from build123d import *

# Parameters (mm, degrees)
BOSS_EXTRUDE1_DEPTH      = 6
BOSS_EXTRUDE1_DEPTH_BACK = 4
SKETCH1_R                = 2.55
SKETCH1_R_2              = 2.2
SKETCH4_W                = 10
SKETCH4_H                = 10
BOSS_EXTRUDE4_DEPTH      = 10
SKETCH5_W                = 4
SKETCH5_H                = 10
CUT_EXTRUDE1_DEPTH       = 10
BOSS_EXTRUDE5_REACH      = 54.82
SKETCH6_R                = 2
CHAMFER1_SIZE            = 2
SKETCH7_W                = 50
SKETCH7_H                = 20.5
BOSS_EXTRUDE6_DEPTH      = 10
SKETCH13_W               = 50
SKETCH13_H               = 10
BOSS_EXTRUDE9_DEPTH      = 25.5
SKETCH16_W               = 44
SKETCH16_H               = 40
CUT_EXTRUDE3_DEPTH       = 7
SKETCH17_R               = 2.6
CUT_EXTRUDE4_DEPTH       = 3
SKETCH18_W               = 2
SKETCH18_H               = 10
BOSS_EXTRUDE11_DEPTH     = 5
FILLET2_R                = 5
CUT_EXTRUDE5_REACH       = 67.666
SKETCH20_R               = 2.55
FILLET5_R                = 1.5
CUT_EXTRUDE6_DEPTH       = 3
BOSS_EXTRUDE12_START     = 2
SKETCH22_W               = 20
SKETCH22_H               = 10
BOSS_EXTRUDE12_DEPTH     = 2
CUT_EXTRUDE7_REACH       = 69.941
SKETCH23_R               = 1.6
CUT_EXTRUDE8_DEPTH       = 68.941151006


with BuildPart() as part:
    # Sketch1 → Boss-Extrude1 (new, two sides: drawn at the far end of the back side and taken through both)
    with BuildSketch(Plane.XY.offset(-BOSS_EXTRUDE1_DEPTH_BACK)):
        Polygon((-15, 0), (-15, 46), (0, 46), (0, 26), (15, 26), (15, 0), align=None)
        with Locations((-7.5, 38.5)):
            Circle(SKETCH1_R, mode=Mode.SUBTRACT)
        with Locations((7.5, 14)):
            Circle(SKETCH1_R_2, mode=Mode.SUBTRACT)
    extrude(amount=BOSS_EXTRUDE1_DEPTH + BOSS_EXTRUDE1_DEPTH_BACK)

    # Sketch4 → Boss-Extrude4 (add)
    with BuildSketch(Plane(origin=(0, 0, -4), x_dir=(-1, 0, 0), z_dir=(0, 0, -1))):
        with Locations((-20, 5)):
            Rectangle(SKETCH4_W, SKETCH4_H)
    extrude(amount=-BOSS_EXTRUDE4_DEPTH)

    # Sketch5 → Cut-Extrude1 (cut)
    with BuildSketch(Plane(origin=(25, 0, 0), x_dir=(0, 0, -1), z_dir=(1, 0, 0))):
        with Locations((-1, 5)):
            Rectangle(SKETCH5_W, SKETCH5_H)
    extrude(amount=-CUT_EXTRUDE1_DEPTH, mode=Mode.SUBTRACT)

    # Sketch6 → Boss-Extrude5 (add, up to next)
    with BuildSketch(Plane.XY.offset(-1), mode=Mode.PRIVATE) as boss_extrude5_sk1:
        with Locations(Location((20, 5, 0), (0, 0, 90))):
            Circle(SKETCH6_R)
    boss_extrude5_tool1 = extrude(boss_extrude5_sk1.sketch, amount=BOSS_EXTRUDE5_REACH, mode=Mode.PRIVATE) - part.part
    add(boss_extrude5_tool1.solids().sort_by_distance((20, 5, -1))[0])

    # Chamfer1
    chamfer1_edges = [part.edges().sort_by_distance(p)[0] for p in [
        (15, 26, 1),
    ]]
    chamfer(chamfer1_edges, length=CHAMFER1_SIZE)

    # Sketch7 → Boss-Extrude6 (add)
    with BuildSketch(Plane.XZ):
        with Locations((5, -4.25)):
            Rectangle(SKETCH7_W, SKETCH7_H)
    extrude(amount=BOSS_EXTRUDE6_DEPTH)

    # Sketch13 → Boss-Extrude9 (add)
    with BuildSketch(Plane(origin=(0, 0, -14.5), x_dir=(-1, 0, 0), z_dir=(0, 0, -1))):
        with Locations((-5, -5)):
            Rectangle(SKETCH13_W, SKETCH13_H)
    extrude(amount=BOSS_EXTRUDE9_DEPTH)

    # Sketch16 → Cut-Extrude3 (cut)
    with BuildSketch(Plane.XZ.offset(10)):
        with Locations((5, -17)):
            Rectangle(SKETCH16_W, SKETCH16_H)
    extrude(amount=-CUT_EXTRUDE3_DEPTH, mode=Mode.SUBTRACT)

    # Sketch17 → Cut-Extrude4 (cut)
    with BuildSketch(Plane.XY.offset(6)):
        with Locations((24.4, -5.6)):
            Circle(SKETCH17_R)
    extrude(amount=-CUT_EXTRUDE4_DEPTH, mode=Mode.SUBTRACT)

    # Sketch18 → Boss-Extrude11 (add)
    with BuildSketch(Plane.ZY.offset(20)):
        with Locations((-10, -5)):
            Rectangle(SKETCH18_W, SKETCH18_H)
    extrude(amount=BOSS_EXTRUDE11_DEPTH)

    # Fillet2
    fillet2_edges = [part.edges().sort_by_distance(p)[0] for p in [
        (-20, -5, -11),
    ]]
    fillet(fillet2_edges, radius=FILLET2_R - 0.0001)  # a hair under: the kernel refuses the full size

    # Sketch19 → Revolve1 (revolve)
    with BuildSketch(Plane.ZY.offset(7.5), mode=Mode.PRIVATE) as revolve1_sk:
        Polygon((-4, 38.5), (-14, 38.5), (-14, 41), (-11.5, 43.5), (-4, 43.5), align=None)
    revolve(revolve1_sk.sketch.rotate(Axis((-7.5, 38.5, -4), (0, 0, -1)), 90), axis=Axis((-7.5, 38.5, -4), (0, 0, -1)))

    # Sketch20 → Cut-Extrude5 (cut, up to next)
    with BuildSketch(Plane.XY.offset(-4), mode=Mode.PRIVATE) as cut_extrude5_sk1:
        with Locations((-7.5, 38.5)):
            Circle(SKETCH20_R)
    cut_extrude5_tool1 = extrude(cut_extrude5_sk1.sketch, amount=-CUT_EXTRUDE5_REACH, mode=Mode.PRIVATE) & part.part
    add(cut_extrude5_tool1.solids().sort_by_distance((-7.5, 38.5, -4))[0], mode=Mode.SUBTRACT)

    # Fillet5
    fillet5_edges = [part.edges().sort_by_distance(p)[0] for p in [
        (-12.5, 38.5, -4),
    ]]
    fillet(fillet5_edges, radius=FILLET5_R)

    # Sketch12 → Cut-Extrude6 (cut)
    with BuildSketch(Plane(origin=(0, 0, 0), x_dir=(1, 0, 0), z_dir=(0, 1, 0))):
        with BuildLine():
            Line((-10.75, 10.5), (-5.75, 10.5))
            ThreePointArc((-5.75, 10.5), (-4.25, 9), (-5.75, 7.5))
            Line((-5.75, 7.5), (-10.75, 7.5))
            ThreePointArc((-10.75, 7.5), (-12.25, 9), (-10.75, 10.5))
        make_face()
    extrude(amount=-CUT_EXTRUDE6_DEPTH, mode=Mode.SUBTRACT)

    # Sketch22 → Boss-Extrude12 (add)
    # profile 1 of 2: a face of its own
    with BuildSketch(Plane(origin=(0, 0, 0), x_dir=(1, 0, 0), z_dir=(0, 1, 0)).offset(BOSS_EXTRUDE12_START)):
        with Locations((-8.25, 9)):
            Rectangle(SKETCH22_W, SKETCH22_H)
        with BuildLine():
            Line((-10.75, 7.5), (-5.75, 7.5))
            ThreePointArc((-5.75, 7.5), (-4.25, 9), (-5.75, 10.5))
            Line((-5.75, 10.5), (-10.75, 10.5))
            ThreePointArc((-10.75, 10.5), (-12.25, 9), (-10.75, 7.5))
        make_face(mode=Mode.SUBTRACT)
    # profile 2 of 2: a face of its own
    with BuildSketch(Plane(origin=(0, 0, 0), x_dir=(1, 0, 0), z_dir=(0, 1, 0)).offset(BOSS_EXTRUDE12_START)):
        with Locations((-8.25, 35)):
            Rectangle(SKETCH22_W, SKETCH22_H)
        with BuildLine():
            Line((-10.75, 36.5), (-5.75, 36.5))
            ThreePointArc((-5.75, 36.5), (-4.25, 35), (-5.75, 33.5))
            Line((-5.75, 33.5), (-10.75, 33.5))
            ThreePointArc((-10.75, 33.5), (-12.25, 35), (-10.75, 36.5))
        make_face(mode=Mode.SUBTRACT)
    extrude(amount=-BOSS_EXTRUDE12_DEPTH)

    # Sketch23 → Cut-Extrude7 (cut, up to next)
    with BuildSketch(Plane(origin=(0, 0, 0), x_dir=(1, 0, 0), z_dir=(0, 1, 0)), mode=Mode.PRIVATE) as cut_extrude7_sk1:
        with Locations(Location((25.25, 22, 0), (0, 0, 180))):
            Circle(SKETCH23_R)
    cut_extrude7_tool1 = extrude(cut_extrude7_sk1.sketch, amount=-CUT_EXTRUDE7_REACH, mode=Mode.PRIVATE) & part.part
    add(cut_extrude7_tool1.solids().sort_by_distance((25.25, 0, -22))[0], mode=Mode.SUBTRACT)

    # Sketch24 → Cut-Extrude8 (cut, through all)
    with BuildSketch(Plane(origin=(0, 0, 0), x_dir=(1, 0, 0), z_dir=(0, 1, 0))):
        with BuildLine():
            Line((-10.75, 33.5), (-5.75, 33.5))
            ThreePointArc((-5.75, 33.5), (-4.25, 35), (-5.75, 36.5))
            Line((-5.75, 36.5), (-10.75, 36.5))
            ThreePointArc((-10.75, 36.5), (-12.25, 35), (-10.75, 33.5))
        make_face()
    extrude(amount=-CUT_EXTRUDE8_DEPTH, mode=Mode.SUBTRACT)


solid = part.part
Design review of the part built by this model. Coordinates are the model's own, in mm. A direction names the side the tool comes from. Give positions to 0.01 mm unless a question says otherwise; leave off trailing zeros. Loops run counter-clockwise (first coordinate to the right, second up) from the corner with the lowest first, then second, coordinate; pieces in that order, holes last. Notation, with made-up numbers: (78.25, -28.5) - (124.25, -28.5) arc R33 cw to (124.25, 7.5) - close; hole circle Ø7 at (-4, -2). An arc over 180 degrees is marked (long way). Write item = value, one per line.
1) Take a section at B-B on z = -35. State the section outline as (x, y) points.
Result sheet:
outline = (-20, -10) - (-17, -10) - (-17, -3) - (-12.25, -3) - (-12.25, 2) - (-18.25, 2) - (-18.25, 0) - (-20, 0) - close; (-4.25, -3) - (27, -3) - (27, -10) - (30, -10) - (30, 0) - (1.75, 0) - (1.75, 2) - (-4.25, 2) - close
2) Tool access review of faces 5 (the face through (25, 5, 4)), 6 (the face through (-8, 1, -14)), 7 (the face through (-8, 2, -7)), 8 (the face through (27, -7, -17)), 9 (the face through (1.75, 1, -9)): name each direction out of +Z, -Z, +X, -X, +Y, -Y from which nothing blocks a thin tool from reaching the whole face with its end or side.
Result sheet:
face_5 = +Z, -Z, +X, +Y
face_6 = +X, -X, +Y
face_7 = -Z, +X, -X
face_8 = -Y
face_9 = -Z, +X, +Y
3) Clearance check with flat-ended pins moving along their axes: pin 1 Ø3 at (y, z) = (-6.5, -23.5) entering from -X; pin 2 Ø5 at (x, z) = (5.5, 0.5) entering from +Y; pin 3 Ø1.6 at (y, z) = (1, -8.5) entering from +X. State where each tip first meets the part, or that it passes through.
Result sheet:
pin_1 = -20
pin_2 = 26
pin_3 = 1.75
4) Draft analysis for pull direction Y (two halves, no side actions). For faces 1 (the face through (21.8, -5.5, 4.5)), 2 (the face through (14, 25, 1)), 3 (the face through (9.6, 14.66, 0.93)), 4 (the face through (-20, -5, -1)), state which applies: +Y half, -Y half, draft (parallel to the pull), parting line (faces both ways), or undercut.
Result sheet:
face_1 = undercut
face_2 = +Y half
face_3 = undercut
face_4 = draft
5) To check wall thickness, follow line 1 (Z direction, x = 25.25, y = -1.55); line 2 (X direction, y = -5.6, z = 4.75); line 3 (Y direction, x = -11, z = -11.5). State the ranges of each line that lie inside material, in increasing order.
Result sheet:
line_1 = -40 to -23.6, -20.4 to 6
line_2 = -20 to 21.8, 27 to 30
line_3 = -3 to 2, 34.93 to 42.07
6) Take a section at C-C on y = 5. State the section outline as (x, z) points.
Result sheet:
outline = (-15, -4) - (25, -4) - (25, -1) - (22, -1) - (22, 3) - (25, 3) - (25, 6) - (-15, 6) - close; hole (15, -1) - (18, -1) - (18, 3) - (15, 3) - close
7) Take a section at A-A on x = 20. State the section outline as (y, z) points, and give its area (3 significant figures).
Result sheet:
outline = (-10, -40) - (0, -40) - (0, -4) - (10, -4) - (10, -1) - (7, -1) - (7, 3) - (10, 3) - (10, 6) - (-10, 6) - (-10, 3) - (-3, 3) - (-3, -37) - (-10, -37) - close; hole (0, -1) - (3, -1) - (3, 3) - (0, 3) - close
area = 256 mm2
8) Take a section at D-D on x = 1. State the section outline as (y, z) points, and give its area (3 significant figures).
Result sheet:
outline = (-10, -40) - (2, -40) - (2, -30) - (0, -30) - (0, -14) - (2, -14) - (2, -4) - (26, -4) - (26, 6) - (-10, 6) - (-10, 3) - (-3, 3) - (-3, -37) - (-10, -37) - close
area = 480 mm2
